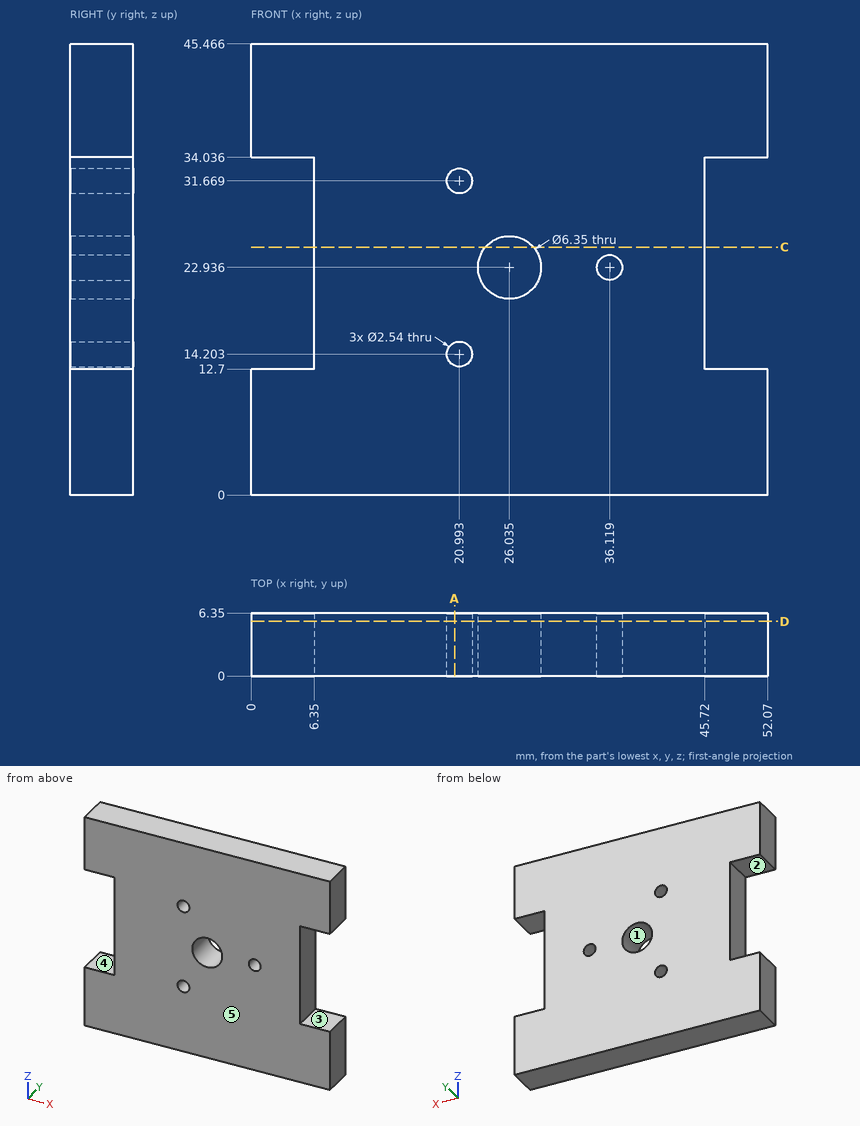
Geometry check sheet. Reference: drawing and pictorial views, mm from the part's lowest x, y, z. A direction names the side the tool comes from. Round coordinates to 2 decimals unless told otherwise and drop trailing zeros. Write each loop counter-clockwise with the first axis right and the second up, starting at its lowest first coordinate (ties: lowest second). Pieces come first, ordered by that corner, then holes.
Item 1: Section check C-C (z = 25). Record the boundary of the cut face in (x, y).
Determined:
outline: (6.35, 0) - (23.62, 0) - (23.62, 6.35) - (6.35, 6.35) - close; (28.45, 0) - (45.72, 0) - (45.72, 6.35) - (28.45, 6.35) - close
Item 2: Mould release check, pull along X, two halves, no side actions. Record for the marked faces 1 and 2: +X half, -X half, draft (parallel to the pull), parting line (faces both ways), or undercut.
Determined:
face 1: undercut
face 2: draft
Item 3: Go/stop test with a flat-tipped pin: pin 1 Ø2 at (y, z) = (3, 26) entering from -X. Record where the tip stops, or that it passes through.
Determined:
pin 1: stops at x = 6.35
Item 4: Access from +Z, -Z, +X, -X, +Y, -Y to the whole of each face (thin tool, end or side, straight path). Record for the marked faces 3, 4 and 5.
Determined:
face 3: +X, +Y, -Y
face 4: -X, +Y, -Y
face 5: +Z, -Z, +X, -X, -Y
Item 5: Material ranges on line 1 along Z through (x, y) = (47.5, 3.75); line 2 along X through (y, z) = (2.5, 23.5); line 3 along X through (y, z) = (1.25, 29), recorded low to high.
Determined:
line 1: z = 0 to 12.7, 34.04 to 45.47
line 2: x = 6.35 to 22.91, 29.16 to 34.98, 37.26 to 45.72
line 3: x = 6.35 to 45.72
Item 6: Section check A-A (x = 20.5). Record the boundary of the cut face in (y, z).
Determined:
outline: (0, 0) - (6.35, 0) - (6.35, 13.03) - (0, 13.03) - close; (0, 15.37) - (6.35, 15.37) - (6.35, 30.5) - (0, 30.5) - close; (0, 32.84) - (6.35, 32.84) - (6.35, 45.47) - (0, 45.47) - close
Item 7: Section check D-D (y = 5.5). Give the number of separate pieces and of enclosed holes in the cut face, plus the area to 3 significant figures.
Determined:
separate pieces: 1
enclosed holes: 4
area: 2,050 mm2
